Autodesk Inventor part; units mm, degrees
ref_plane "YZ Plane" through (0, 0, 0) normal (1, 0, 0) x (0, 1, 0)
ref_plane "XZ Plane" through (0, 0, 0) normal (0, 1, 0) x (-1, 0, 0)
ref_plane "XY Plane" through (0, 0, 0) normal (0, 0, 1) x (1, 0, 0)
sketch "Sketch1" plane through (0, 0, 0) normal (0, 0, 1) x (1, 0, 0)
  line L0 (-20, 20) -> (20, 20)
  line L1 (20, 20) -> (20, -20)
  line L2 (20, -20) -> (-20, -20)
  line L3 (-20, -20) -> (-20, 20)
  line L4 (-20, 20) -> (20, -20) construction
  line L5 (20, 20) -> (-20, -20) construction
  point P0 (0, 0)
  dimension "d0" = 40
  dimension "d1" = 40
extrude "Extrusion1" add sketch "Sketch1" along normal mid plane 47
sketch "Sketch2" plane through (0, 0, 23.5) normal (0, 0, 1) x (1, 0, 0)
  circle A0 centre (0, 0) radius 2.5
  dimension "d4" = 5
extrude "Extrusion2" add sketch "Sketch2" along normal blind 25
sketch "Sketch3" plane through (0, 0, 23.5) normal (0, 0, 1) x (1, 0, 0)
  circle A0 centre (0, 0) radius 11
  dimension "d7" = 22
extrude "Extrusion3" add sketch "Sketch3" along normal blind 2.5
properties part number "NEMA 17 PARA TAPA PRINCIPAL"
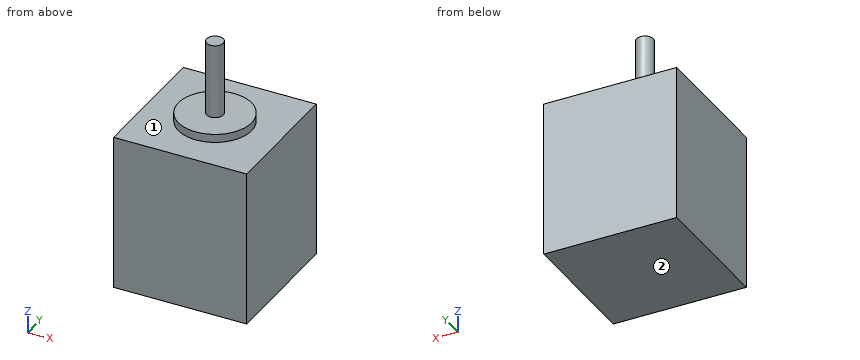
Work out the finished part from the listing and answer in its coordinate system (mm). Face numbers are marked on the shaded views. A direction names the side the tool comes from. Round coordinates to 2 decimals unless told otherwise and drop trailing zeros. Write each loop counter-clockwise with the first axis right and the second up, starting at its lowest first coordinate (ties: lowest second). Pieces come first, ordered by that corner, then holes.
1) A cutting plane is placed at A-A on y = 0. Determine the outline of the cut face in (x, z).
2) A cutting plane is placed at D-D on y = 6.5. Determine the outline of the cut face in (x, z).
3) Consider probe 1 along Z at (x, y) = (15, 5); probe 2 along Z at (x, y) = (6.5, 7.5). Determine where each line is inside the solid, lowest interval first.
4) A cutting plane is placed at C-C on z = 37.5. Determine the outline of the cut face in (x, y).
5) Which of the six approach directions +Z, -Z, +X, -X, +Y, -Y give full straight-line access (tool end or side, diameter ignored) to the marked faces 1 and 2?
6) Flat-ended cylindrical pins translate along their axes: P1, Ø11, axis at x = 1.5, y = 4.5, coming from the +Z side; P2, Ø2, axis at x = -6.5, y = -6.5, coming from the +Z side; P3, Ø2, axis at x = -1, z = 32, coming from the -Y side. Find the tip coordinate at first contact, or state that the pin passes through.
Entries:
1. outline: (-20, -23.5) - (20, -23.5) - (20, 23.5) - (11, 23.5) - (11, 26) - (2.5, 26) - (2.5, 48.5) - (-2.5, 48.5) - (-2.5, 26) - (-11, 26) - (-11, 23.5) - (-20, 23.5) - close
2. outline: (-20, -23.5) - (20, -23.5) - (20, 23.5) - (8.87, 23.5) - (8.87, 26) - (-8.87, 26) - (-8.87, 23.5) - (-20, 23.5) - close
3. probe 1: z = -23.5 to 23.5
3. probe 2: z = -23.5 to 26
4. outline: circle Ø5 at (0, 0)
5. face 1: +Z
5. face 2: -Z, +X, -X, +Y, -Y
6. P1: stops at z = 48.5
6. P2: stops at z = 26
6. P3: stops at y = -2.5
